The model under review builds one solid part; all positions refer to its coordinate system, in mm. Face numbers are marked on the shaded views. Give positions to 0.01 mm unless a question says otherwise; leave off trailing zeros. Write each loop counter-clockwise with the first axis right and the second up, starting at its lowest first coordinate (ties: lowest second). Pieces come first, ordered by that corner, then holes. Notation, with made-up numbers: (40.25, 61.5) - (85.25, 61.5) arc R28 cw to (85.25, 88.5) - close; hole circle Ø9 at (-5.75, -23.75). An arc over 180 degrees is marked (long way). Write item = value, one per line.
```python
from build123d import *
from build123d.topology import SkipClean

# Parameters (mm, degrees)
SKETCH1_R                = 3.5
SKETCH1_R_2              = 2.5
BOSS_EXTRUDE1_DEPTH      = 3
SKETCH2_R                = 3.5
BOSS_EXTRUDE2_DEPTH      = 1
CUT_EXTRUDE1_REACH       = 8.364
SKETCH3_R                = 1.3
SKETCH4_R                = 3.5
SKETCH4_R_2              = 2.4
BOSS_EXTRUDE3_DEPTH      = 3
CHAMFER1_SIZE            = 0.5
BOSS_EXTRUDE5_DEPTH      = 3.5
BOSS_EXTRUDE5_DEPTH_BACK = 3
FILLET1_R                = 0.5
BOSS_EXTRUDE6_START      = 3
BOSS_EXTRUDE6_DEPTH      = 3
CUT_EXTRUDE2_START       = -4
CUT_EXTRUDE2_DEPTH       = 4
FILLET3_R                = 0.5


# Some blends are built 0.0001 mm under size
with BuildPart() as part:
    # Sketch1 → Boss-Extrude1 (new body)
    with BuildSketch(Plane(origin=(0, 0, 0), x_dir=(1, 0, 0), z_dir=(0, 1, 0))):
        with Locations(Location((0, 0, 0), (0, 0, 270))):
            Circle(SKETCH1_R)
        with Locations(Location((0, 0, 0), (0, 0, 270))):
            Circle(SKETCH1_R_2, mode=Mode.SUBTRACT)
    extrude(amount=BOSS_EXTRUDE1_DEPTH)

    # Sketch2 → Boss-Extrude2 (add)
    with BuildSketch(Plane(origin=(0, 3, 0), x_dir=(1, 0, 0), z_dir=(0, 1, 0))):
        with Locations(Location((0, 0, 0), (0, 0, 270))):
            Circle(SKETCH2_R)
    extrude(amount=BOSS_EXTRUDE2_DEPTH)

    # Sketch3 → Cut-Extrude1 (cut, up to next)
    with BuildSketch(Plane(origin=(0, 4, 0), x_dir=(1, 0, 0), z_dir=(0, 1, 0)), mode=Mode.PRIVATE) as cut_extrude1_sk1:
        with Locations(Location((0, 0, 0), (0, 0, 270))):
            Circle(SKETCH3_R)
    cut_extrude1_tool1 = extrude(cut_extrude1_sk1.sketch, amount=-CUT_EXTRUDE1_REACH, mode=Mode.PRIVATE) & part.part
    add(cut_extrude1_tool1.solids().sort_by_distance((0, 4, 0))[0], mode=Mode.SUBTRACT)

    # Sketch4 → Boss-Extrude3 (add)
    with BuildSketch(Plane(origin=(0, 4, 0), x_dir=(1, 0, 0), z_dir=(0, 1, 0))):
        with Locations(Location((0, 0, 0), (0, 0, 270))):
            Circle(SKETCH4_R)
        with Locations(Location((0, 0, 0), (0, 0, 270))):
            Circle(SKETCH4_R_2, mode=Mode.SUBTRACT)
    extrude(amount=BOSS_EXTRUDE3_DEPTH)

    # Chamfer1
    chamfer1_edges = [part.edges().sort_by_distance(p)[0] for p in [
        (0, 7, -2.4),
        (0, 0, -2.5),
    ]]
    chamfer(chamfer1_edges, length=CHAMFER1_SIZE)

    # Sketch6 → Boss-Extrude5 (add, two sides: drawn at the far end of the back side and taken through both)
    with BuildSketch(Plane(origin=(0, 3.5, 0), x_dir=(1, 0, 0), z_dir=(0, 1, 0)).offset(-BOSS_EXTRUDE5_DEPTH_BACK)):
        with BuildLine():
            Line((-25, 12.385879056), (-3.136200717, 1.553784111))
            ThreePointArc((-3.136200717, 1.553784111), (0, 3.5), (3.136200717, 1.553784111))
            Line((3.136200717, 1.553784111), (25, 12.385879056))
            ThreePointArc((25, 12.385879056), (0, 27.9), (-25, 12.385879056))
        make_face()
    extrude(amount=BOSS_EXTRUDE5_DEPTH + BOSS_EXTRUDE5_DEPTH_BACK)

    # Fillet1
    fillet1_edges = [part.edges().sort_by_distance(p)[0] for p in [
        (-2.973906891, 7, 1.845502047),
        (0, 0.5, -3.5),
    ]]
    fillet(fillet1_edges, radius=FILLET1_R - 0.0001)  # a hair under: the kernel refuses the full size

    # Sketch7 → Boss-Extrude6 (add)
    with BuildSketch(Plane.XZ.offset(-0.5).offset(BOSS_EXTRUDE6_START)):
        with BuildLine():
            Line((25, -12.385879056), (12.096774194, -5.993167285))
            ThreePointArc((12.096774194, -5.993167285), (0, -13.5), (-12.096774194, -5.993167285))
            Line((-12.096774194, -5.993167285), (-25, -12.385879056))
            ThreePointArc((-25, -12.385879056), (0, -27.9), (25, -12.385879056))
        make_face()
    extrude(amount=-BOSS_EXTRUDE6_DEPTH)

    # Sketch8 → Cut-Extrude2 (cut)
    with SkipClean():  # the faces are left unmerged after this step: merging them gives an invalid solid
        with BuildSketch(Plane(origin=(0, 7, 0), x_dir=(1, 0, 0), z_dir=(0, 1, 0)).offset(CUT_EXTRUDE2_START)):
            with BuildLine():
                Line((3.136200717, 1.553784111), (25, 12.385879056))
                ThreePointArc((25, 12.385879056), (0, 27.9), (-25, 12.385879056))
                Line((-25, 12.385879056), (-3.136200717, 1.553784111))
                ThreePointArc((-3.136200717, 1.553784111), (0, 3.5), (3.136200717, 1.553784111))
            make_face()
        extrude(amount=CUT_EXTRUDE2_DEPTH, mode=Mode.SUBTRACT)

    # Fillet3
    # the kernel refuses this fillet: 0.5 mm, written as the material it takes off along each edge
    with BuildSketch(Plane(origin=(0, 7, 0), x_dir=(-0.8960573476702508, 0, -0.44393831743402734), z_dir=(-0.44393831743402734, 0, 0.8960573476702508))) as fillet3_piece_1:
        with BuildLine():
            CenterArc((3.5 - FILLET3_R, FILLET3_R), FILLET3_R, 270, 90)
            Line((3.5, FILLET3_R), (3.5 + FILLET3_R * 0.02, FILLET3_R))
            Line((3.5 + FILLET3_R * 0.02, FILLET3_R), (3.5 + FILLET3_R * 0.02, -FILLET3_R * 0.02))
            Line((3.5 + FILLET3_R * 0.02, -FILLET3_R * 0.02), (3.5 - FILLET3_R, -FILLET3_R * 0.02))
            Line((3.5 - FILLET3_R, -FILLET3_R * 0.02), (3.5 - FILLET3_R, 0))
        make_face()
    revolve(axis=Axis((0, 7, 0), (0, -1, 0)), revolution_arc=127.289134778, mode=Mode.SUBTRACT)


solid = part.part
```
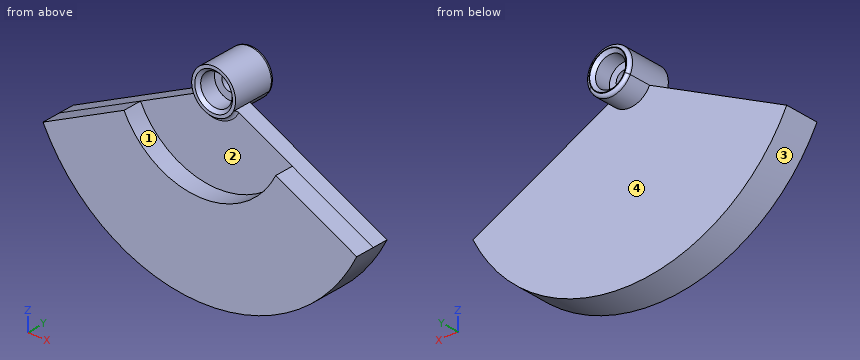
1. Draft analysis for pull direction X (two halves, no side actions). For the marked faces 1, 2, 3 and 4, state which applies: +X half, -X half, draft (parallel to the pull), parting line (faces both ways), or undercut.
Findings below:
face_1 = undercut
face_2 = undercut
face_3 = parting line
face_4 = draft
2. Take a section at D-D on x = -11. Give the boundary of the cut face in (y, z).
Findings below:
outline = (-2.5, -25.64) - (3, -25.64) - (3, -5.45) - (0.5, -5.45) - (0.5, -7.83) - (-2.5, -7.83) - close
3. Insertion check: P1, Ø2.5, axis at x = 0, z = -1, coming from the -Y side; P2, Ø8, axis at x = -1.5, z = -11.5, coming from the +Y side; P3, Ø5.5, axis at x = 0, z = 0, coming from the -Y side. Each pin has a flat end and moves straight along its axis. Give the tip position at first contact, or say it passes through.
Findings below:
P1 = 3
P2 = 3
P3 = 0.25
4. For line 1 (X direction, y = 3.65, z = 0); line 2 (X direction, y = 2.3, z = 0); line 3 (Y direction, x = 19, z = -15.5), list the stretches that pass through material, from the lowest coordinate up. Write a range as from..to.
Findings below:
line_1 = -3.5..-1.3, 1.3..3.5
line_2 = -3.5..-2.5, 2.5..3.5
line_3 = -2.5..3
5. Take a section at C-C on y = 1.25. Give the boundary of the cut face in (x, z), and give its area (3 significant figures).
Findings below:
outline = (-25, -12.39) arc R27.9 ccw to (25, -12.39) - (3.14, -1.55) arc R3.5 ccw (long way) to (-3.14, -1.55) - close; hole circle Ø5 at (0, 0)
area = 870 mm²
6. Take a section at B-B on z = 0. Give the boundary of the cut face in (x, y), and give its area (3 significant figures).
Findings below:
outline = (-3.5, 0) - (-3, 0) - (-2.5, 0.5) - (-2.5, 3) - (-1.3, 3) - (-1.3, 4) - (-2.4, 4) - (-2.4, 6.5) - (-2.9, 7) - (-3, 7) arc R0.5 ccw to (-3.5, 6.5) - close; (1.3, 3) - (2.5, 3) - (2.5, 0.5) - (3, 0) - (3.5, 0) - (3.5, 6.5) arc R0.5 ccw to (3, 7) - (2.9, 7) - (2.4, 6.5) - (2.4, 4) - (1.3, 4) - close
area = 16.4 mm²
